Design review of the part shown in the three views and the two pictorial views. Dimensions are in mm from the part's minimum x, y and z. A direction names the side the tool comes from. Give positions to 0.01 mm unless a question says otherwise; leave off trailing zeros. Write each loop counter-clockwise with the first axis right and the second up, starting at its lowest first coordinate (ties: lowest second). Pieces come first, ordered by that corner, then holes. Notation, with made-up numbers: (49, 51) -> (104, 51) arc R21 ccw to (104, 67) -> close; hole circle Ø6 at (40.5, 1.25). An arc over 180 degrees is marked (long way). Use CSV: the item, a comma, the result in double quotes.
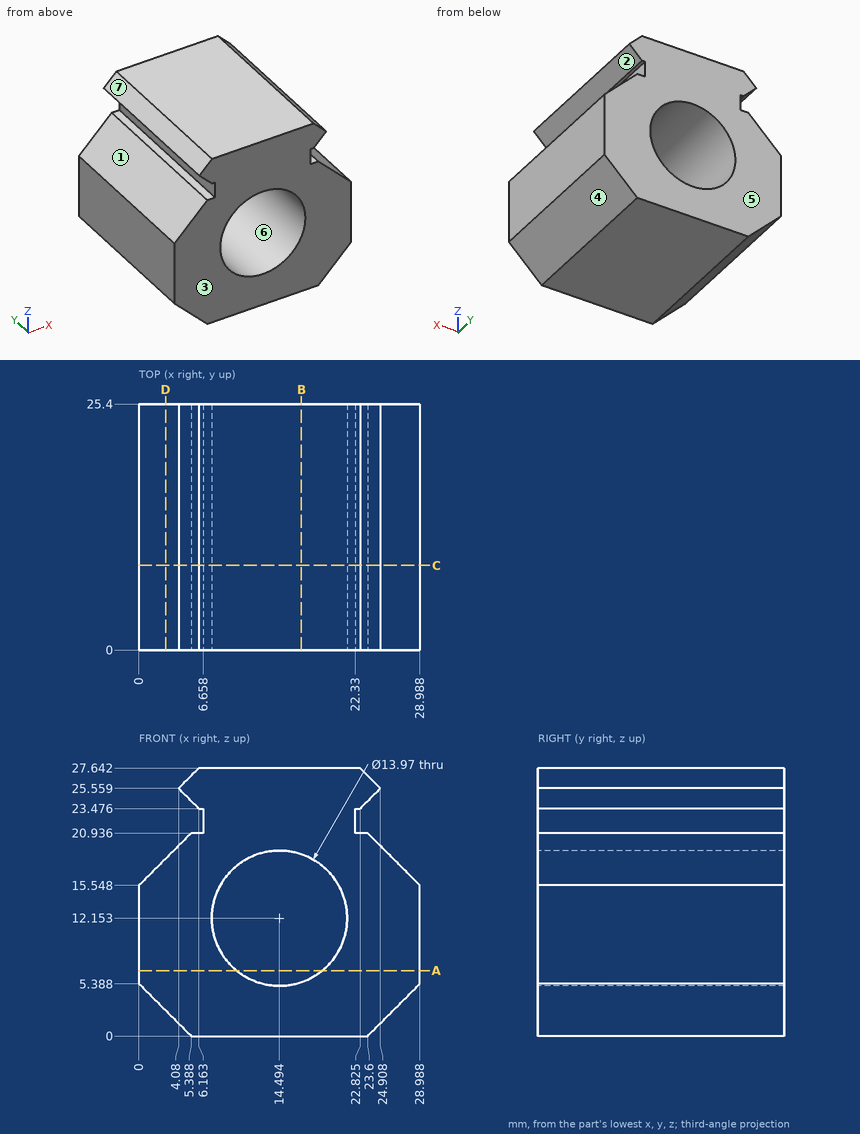
Q1. Insertion check: pin 1 (1.3 mm diameter, centred on y = 15.5, z = 22.5, fed in from +X); pin 2 (8 mm diameter, centred on x = 19.5, z = 9.5, fed in from -Y); pin 3 (8 mm diameter, centred on x = 16.5, z = 11.5, fed in from -Y); pin 4 (8 mm diameter, centred on y = 6, z = 24.5, fed in from -X). Each pin has a flat end and moves straight along its axis. Give the tip position at first contact, or say it passes through.
Derived:
pin 1,"stops at x = 22.33"
pin 2,"stops at y = 0"
pin 3,"passes through"
pin 4,"stops at x = 4.08"
Q2. The part is to be moulded in two halves that separate along Z. For the marked faces 4, 5, 6 and 7, say which applies: pulls with the +Z half, pulls with the -Z half, needs draft (parallel to the pull), parting line crosses it, or undercut.
Derived:
face 4,"pulls with the -Z half"
face 5,"needs draft"
face 6,"undercut"
face 7,"pulls with the +Z half"
Q3. Consider section A-A (z = 6.75). Write out the cut boundary in (x, y).
Derived:
outline,"(0, 0) -> (10.07, 0) -> (10.07, 25.4) -> (0, 25.4) -> close; (18.92, 0) -> (28.99, 0) -> (28.99, 25.4) -> (18.92, 25.4) -> close"
Q4. Machinability: for the marked faces 1, 2 and 3, which of the approach directions +Z, -Z, +X, -X, +Y, -Y give a long, thin tool a straight path to every point of the face, cutting with its end or side? Answer none if there is none.
Derived:
face 1,"-X, +Y, -Y"
face 2,"+X, +Y, -Y"
face 3,"+Z, -Z, +X, -X, -Y"
Q5. Consider section B-B (x = 16.75). Write out the cut boundary in (y, z).
Derived:
outline,"(0, 0) -> (25.4, 0) -> (25.4, 5.54) -> (0, 5.54) -> close; (0, 18.76) -> (25.4, 18.76) -> (25.4, 27.64) -> (0, 27.64) -> close"
Q6. Consider section D-D (x = 2.75). Write out the cut boundary in (y, z), then the cut area to 3 significant figures.
Derived:
outline,"(0, 2.64) -> (25.4, 2.64) -> (25.4, 18.3) -> (0, 18.3) -> close"
area,"398 mm2"
Q7. Consider section C-C (y = 8.75). Write out the cut boundary in (x, z) (1 decimal).
Derived:
outline,"(0, 5.4) -> (5.4, 0) -> (23.6, 0) -> (29, 5.4) -> (29, 15.5) -> (23.6, 20.9) -> (22.3, 20.9) -> (22.3, 23.5) -> (22.8, 23.5) -> (24.9, 25.6) -> (22.8, 27.6) -> (6.2, 27.6) -> (4.1, 25.6) -> (6.2, 23.5) -> (6.7, 23.5) -> (6.7, 20.9) -> (5.4, 20.9) -> (0, 15.5) -> close; hole circle Ø14 at (14.5, 12.2)"
Q8. To check wall thickness, follow probe 1 along X at (y, z) = (11, 21.25); probe 2 along X at (y, z) = (6, 5.75) (1 decimal); probe 3 along X at (y, z) = (10.25, 9.5) (1 decimal). State the ranges of each line that lie inside material, in increasing order.
Derived:
probe 1,"x = 6.66 to 22.33"
probe 2,"x = 0 to 11.7, 17.3 to 29"
probe 3,"x = 0 to 8, 21 to 29"
